from build123d import *

# Parameters (mm, degrees)
SKETCH_1_R          = 17.5
SKETCH_1_R_2        = 12
EXTRUDE_1_DEPTH     = 2636
SKETCH_2_R          = 12.6
CUT_EXTRUDE_1_DEPTH = 52
SKETCH_3_R          = 12.6
CUT_EXTRUDE_2_DEPTH = 52
CUT_EXTRUDE_3_DEPTH = 20
CUT_EXTRUDE_4_DEPTH = 20


with BuildPart() as part:
    # 草图1 → 凸台-拉伸1 (new body)
    with BuildSketch(Plane(origin=(0, 0, 0), x_dir=(0, 0, -1), z_dir=(1, 0, 0))):
        Circle(SKETCH_1_R)
        Circle(SKETCH_1_R_2, mode=Mode.SUBTRACT)
    extrude(amount=EXTRUDE_1_DEPTH)

    # 草图2 → 切除-拉伸1 (cut)
    with BuildSketch(Plane.ZY):
        Circle(SKETCH_2_R)
    extrude(amount=-CUT_EXTRUDE_1_DEPTH, mode=Mode.SUBTRACT)

    # 草图3 → 切除-拉伸2 (cut)
    with BuildSketch(Plane(origin=(2636, 0, 0), x_dir=(0, 0, -1), z_dir=(1, 0, 0))):
        Circle(SKETCH_3_R)
    extrude(amount=-CUT_EXTRUDE_2_DEPTH, mode=Mode.SUBTRACT)

    # 草图4 → 切除-拉伸3 (cut, symmetric)
    with BuildSketch(Plane.XY):
        with BuildLine():
            Line((20, 3), (25, 3))
            ThreePointArc((25, 3), (28, 0), (25, -3))
            Line((25, -3), (20, -3))
            ThreePointArc((20, -3), (17, 0), (20, 3))
        make_face()
    extrude(amount=CUT_EXTRUDE_3_DEPTH, both=True, mode=Mode.SUBTRACT)

    # 草图5 → 切除-拉伸4 (cut, symmetric)
    with BuildSketch(Plane.XY):
        with BuildLine():
            Line((2611, 3), (2616, 3))
            ThreePointArc((2616, 3), (2619, 0), (2616, -3))
            Line((2616, -3), (2611, -3))
            ThreePointArc((2611, -3), (2608, 0), (2611, 3))
        make_face()
    extrude(amount=CUT_EXTRUDE_4_DEPTH, both=True, mode=Mode.SUBTRACT)


solid = part.part
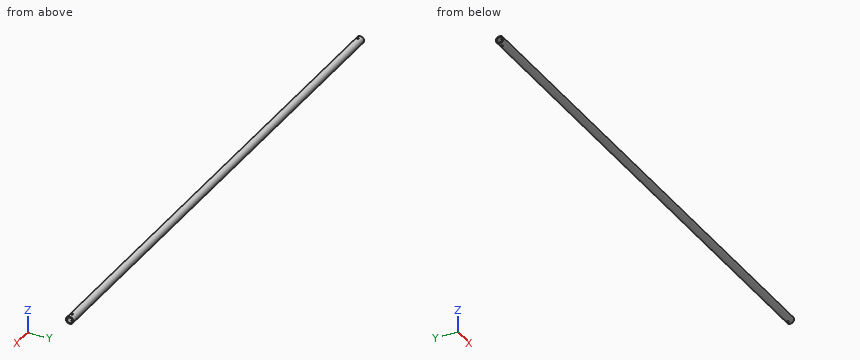
Verification items for the finished model (mm, model axes). Coordinates: 2 decimals unless noted, no trailing zeros. Loops run counter-clockwise (first coordinate to the right, second up) from the corner with the lowest first, then second, coordinate; pieces in that order, holes last. Notation, with made-up numbers: M 88.5,57 L 142.5,57 A31 ccw 142.5,86 Z; hole C -34.5,-26 d1. An arc over 180 degrees is marked long. One line per item, written item: value.
1. Section check A-A on z = 0. Record the cut outline in (x, y), plus the area to 3 significant figures.
Answers follow:
outline: M 0,-17.5 L 2636,-17.5 L 2636,-12.6 L 2584,-12.6 L 2584,-12 L 52,-12 L 52,-12.6 L 0,-12.6 Z; M 0,12.6 L 52,12.6 L 52,12 L 2584,12 L 2584,12.6 L 2636,12.6 L 2636,17.5 L 0,17.5 Z
area: 28,900 mm^2
2. Section check B-B on x = 198.5. Record the cut outline in (y, z).
Answers follow:
outline: C 0,0 d35; hole C 0,0 d24
3. Material ranges on line 1 along X through (y, z) = (1, 16); line 2 along Y through (x, z) = (37, 0); line 3 along Y through (x, z) = (1679, -1), recorded low to high. Write a range as from..to.
Answers follow:
line 1: 0..17.17, 27.83..2608.17, 2618.83..2636
line 2: -17.5..-12.6, 12.6..17.5
line 3: -17.47..-11.96, 11.96..17.47
4. Gauge pin test, flat ends, axial feed: P1, Ø4, axis at x = 2613, z = 16, coming from the +Y side; P2, Ø10, axis at x = 2055, z = -7, coming from the -Y side; P3, Ø1.5, axis at x = 22.5, z = -14, coming from the +Y side. Record the tip position at first contact, or that the pin passes through.
Answers follow:
P1: y = 10.5
P2: y = -17.39
P3: y = 11.43
